Here's how the part is built. I have some questions about the finished solid (model axes, mm). Give positions to 0.01 mm unless a question says otherwise; leave off trailing zeros. Write each loop counter-clockwise with the first axis right and the second up, starting at its lowest first coordinate (ties: lowest second). Pieces come first, ordered by that corner, then holes. Notation, with made-up numbers: (3, 21) -> (15, 21) arc R10 ccw to (15, 38) -> close; hole circle Ø6 at (66, 39.5). An arc over 180 degrees is marked (long way). Put each result on its own line as item: value. Start each with the question number.
from build123d import *

# Parameters (mm, degrees)
SKETCH1_W                     = 2320.925
SKETCH1_H                     = 419.1
BOSS_EXTRUDE1_DEPTH           = 546.1
SKETCH2_R                     = 228.6
BOSS_EXTRUDE2_DEPTH           = 127
BOSS_EXTRUDE2_DRAFT           = 5
BOSS_EXTRUDE2_PROFILE_2_DEPTH = 127
BOSS_EXTRUDE2_PROFILE_2_DRAFT = 5
BOSS_EXTRUDE2_PROFILE_3_DEPTH = 127
BOSS_EXTRUDE2_PROFILE_3_DRAFT = 5


with BuildPart() as part:
    # Sketch1 → Boss-Extrude1 (new body)
    with BuildSketch(Plane(origin=(0, 0, 0), x_dir=(1, 0, 0), z_dir=(0, 1, 0))):
        Rectangle(SKETCH1_W, SKETCH1_H)
    extrude(amount=BOSS_EXTRUDE1_DEPTH)


with BuildPart() as boss_extrude2_tool:
    # Sketch2 → Boss-Extrude2 (with draft: the straight prism first)
    with BuildSketch(Plane.XY.offset(209.55)):
        with Locations((0, 273.05)):
            Circle(SKETCH2_R)
    extrude(amount=BOSS_EXTRUDE2_DEPTH)
    # Boss-Extrude2: the draft: its side faces are tilted about the plane it starts from
    boss_extrude2_sides = [boss_extrude2_tool.faces().sort_by_distance(p)[0] for p in [
        (-228.6, 273.05, 273.05),
    ]]
    draft(boss_extrude2_sides, Plane.XY.offset(209.55), BOSS_EXTRUDE2_DRAFT)


with BuildPart() as part_1:
    add(part.part)

    # Boss-Extrude2: add boss_extrude2_tool
    add(boss_extrude2_tool.part)


with BuildPart() as boss_extrude2_profile_2_tool:
    # Sketch2 → Boss-Extrude2 profile 2 (with draft: the straight prism first)
    with BuildSketch(Plane.XY.offset(209.55)):
        with Locations((779.4625, 273.05)):
            Circle(SKETCH2_R)
    extrude(amount=BOSS_EXTRUDE2_PROFILE_2_DEPTH)
    # Boss-Extrude2 profile 2: the draft: its side faces are tilted about the plane it starts from
    boss_extrude2_profile_2_sides = [boss_extrude2_profile_2_tool.faces().sort_by_distance(p)[0] for p in [
        (550.8625, 273.05, 273.05),
    ]]
    draft(boss_extrude2_profile_2_sides, Plane.XY.offset(209.55), BOSS_EXTRUDE2_PROFILE_2_DRAFT)


with BuildPart() as part_2:
    add(part_1.part)

    # Boss-Extrude2 profile 2: add boss_extrude2_profile_2_tool
    add(boss_extrude2_profile_2_tool.part)


with BuildPart() as boss_extrude2_profile_3_tool:
    # Sketch2 → Boss-Extrude2 profile 3 (with draft: the straight prism first)
    with BuildSketch(Plane.XY.offset(209.55)):
        with Locations((-779.4625, 273.05)):
            Circle(SKETCH2_R)
    extrude(amount=BOSS_EXTRUDE2_PROFILE_3_DEPTH)
    # Boss-Extrude2 profile 3: the draft: its side faces are tilted about the plane it starts from
    boss_extrude2_profile_3_sides = [boss_extrude2_profile_3_tool.faces().sort_by_distance(p)[0] for p in [
        (-1008.0625, 273.05, 273.05),
    ]]
    draft(boss_extrude2_profile_3_sides, Plane.XY.offset(209.55), BOSS_EXTRUDE2_PROFILE_3_DRAFT)


with BuildPart() as part_3:
    add(part_2.part)

    # Boss-Extrude2 profile 3: add boss_extrude2_profile_3_tool
    add(boss_extrude2_profile_3_tool.part)


solid = part_3.part
1) Thinking about a two-plate mould opening in X: for faces 1 (the flat face through (-16, 546.1, -3)), 2 (the flat face through (-16, 27, 209.55)), 3 (the conical face through (-827.563, 56.439, 286.272)), 4 (the flat face through (1160.462, 269, 3)), which applies, released by +X, released by -X, zero draft, split by the parting line, or undercut?
2) I'm going to push a flat-ended pin straight in: pin 1 Ø1.5 at (x, y) = (461.5, 385.5) entering from +Z. Where does the tip first touch, or does it pass through?
3) I want a section at A-A, the plane x = 0. Write out the boundary of the cut face in (y, z).
4) I want a section at B-B, the plane y = 273.05. Write out the boundary of the cut face in (x, z).
5) I need wall thicknesses on probe 1 along X at (y, z) = (262, 231); probe 2 along Z at (x, y) = (871.5, 509); probe 3 along Y at (x, z) = (-89, 212.5). Which ranges of each line are inside material? Lowest first, please.
Established:
1. face 1: zero draft
1. face 2: undercut
1. face 3: undercut
1. face 4: released by +X
2. pin 1: stops at z = 209.55
3. outline: (0, -209.55) -> (546.1, -209.55) -> (546.1, 209.55) -> (501.65, 209.55) -> (490.54, 336.55) -> (55.56, 336.55) -> (44.45, 209.55) -> (0, 209.55) -> close
4. outline: (-1160.46, -209.55) -> (1160.46, -209.55) -> (1160.46, 209.55) -> (1008.06, 209.55) -> (996.95, 336.55) -> (561.97, 336.55) -> (550.86, 209.55) -> (228.6, 209.55) -> (217.49, 336.55) -> (-217.49, 336.55) -> (-228.6, 209.55) -> (-550.86, 209.55) -> (-561.97, 336.55) -> (-996.95, 336.55) -> (-1008.06, 209.55) -> (-1160.46, 209.55) -> close
5. probe 1: x = -1005.92 to -553.01, -226.45 to 226.45, 553.01 to 1005.92
5. probe 2: z = -209.55 to 209.55
5. probe 3: y = 62.77 to 483.33
